Design review of the part built by this model. Coordinates are the model's own, in mm. A direction names the side the tool comes from. Give positions to 0.01 mm unless a question says otherwise; leave off trailing zeros. Order: outer loops, then holes, each group sorted by start corner. A loop starts at its lowest first (then second) coordinate and runs counter-clockwise, first axis right, second up. Notation, with made-up numbers: (45.5, -26) -> (93.5, -26) arc R32 cw to (93.5, 8) -> close; hole circle Ø4 at (-3, 78). An arc over 180 degrees is marked (long way). One line per item, written item: value. Start each with the question number.
1) Consider section A-A (x = 29). State the section outline as (y, z) points.
2) Tool access review of faces 1 (the face through (-40, 4, 0)), 2 (the face through (-37, 7, -26)), 3 (the face through (-1, 4, -27.5)), 4 (the face through (-1, 4, 27.5)), 5 (the face through (35, 3, 0)): name each direction out of +Z, -Z, +X, -X, +Y, -Y from which nothing blocks a thin tool from reaching the whole face with its end or side.
3) For pin 1 (2.5 mm diameter, centred on y = 3, z = 4.5, fed in from +X); pin 2 (1 mm diameter, centred on y = 3.5, z = -16, fed in from +X); pin 3 (3 mm diameter, centred on x = -2, y = 6, fed in from -Z); pin 4 (1 mm diameter, centred on y = 6.5, z = 26.5, fed in from -X), all flat-tipped, find the tip position at first contact; note any pin that passes through.
4) Consider section C-C (x = -55.5). State the section outline as (y, z) points.
5) The part is to be moulded in two halves that separate along X. For faces 6 (the face through (0, 3, 22.5)), 7 (the face through (37, 7, 26)), 8 (the face through (40, 4, 0)), say which applies: released by +X, released by -X, zero draft, split by the parting line, or undercut.
6) Wall thickness on line 1 along X through (y, z) = (1.75, -20); line 2 along X through (y, z) = (5.25, -26); line 3 along Z through (x, y) = (-31.5, 2.25): over which ranges is each line inside the solid? List them lowest first. Write a range as from..to.
7) Consider section B-B (z = 5). State the section outline as (x, y) points, plus the area to 3 significant figures.
from build123d import *

# Parameters (mm, degrees)
SKETCH1_W           = 132
SKETCH1_H           = 87
BOSS_EXTRUDE1_DEPTH = 2
SKETCH2_W           = 80
SKETCH2_H           = 55
BOSS_EXTRUDE2_DEPTH = 5
SKETCH3_W           = 76
SKETCH3_H           = 51
CUT_EXTRUDE1_DEPTH  = 2
CUT_EXTRUDE2_REACH  = 7
SKETCH4_W           = 70
SKETCH4_H           = 45
SKETCH5_W           = 2
SKETCH5_H           = 41
SKETCH5_W_2         = 66
SKETCH5_H_2         = 2
CUT_EXTRUDE3_DEPTH  = 2
CUT_EXTRUDE4_DEPTH  = 2


with BuildPart() as part:
    # Sketch1 → Boss-Extrude1 (new body)
    with BuildSketch(Plane(origin=(0, 0, 0), x_dir=(1, 0, 0), z_dir=(0, 1, 0))):
        Rectangle(SKETCH1_W, SKETCH1_H)
    extrude(amount=BOSS_EXTRUDE1_DEPTH)

    # Sketch2 → Boss-Extrude2 (add)
    with BuildSketch(Plane(origin=(0, 2, 0), x_dir=(1, 0, 0), z_dir=(0, 1, 0))):
        Rectangle(SKETCH2_W, SKETCH2_H)
    extrude(amount=BOSS_EXTRUDE2_DEPTH)

    # Sketch3 → Cut-Extrude1 (cut)
    with BuildSketch(Plane(origin=(0, 7, 0), x_dir=(1, 0, 0), z_dir=(0, 1, 0))):
        Rectangle(SKETCH3_W, SKETCH3_H)
    extrude(amount=-CUT_EXTRUDE1_DEPTH, mode=Mode.SUBTRACT)

    # Sketch4 → Cut-Extrude2 (cut, up to next)
    with BuildSketch(Plane(origin=(0, 5, 0), x_dir=(1, 0, 0), z_dir=(0, 1, 0)), mode=Mode.PRIVATE) as cut_extrude2_sk1:
        Rectangle(SKETCH4_W, SKETCH4_H)
    cut_extrude2_tool1 = extrude(cut_extrude2_sk1.sketch, amount=-CUT_EXTRUDE2_REACH, mode=Mode.PRIVATE) & part.part
    add(cut_extrude2_tool1.solids().sort_by_distance((0, 5, 0))[0], mode=Mode.SUBTRACT)

    # Sketch5 → Cut-Extrude3 (cut)
    with BuildSketch(Plane(origin=(0, 7, 0), x_dir=(1, 0, 0), z_dir=(0, 1, 0))):
        with Locations((-39, 0)):
            Rectangle(SKETCH5_W, SKETCH5_H)
        with Locations((39, 0)):
            Rectangle(SKETCH5_W, SKETCH5_H)
        with Locations((0, 26.5)):
            Rectangle(SKETCH5_W_2, SKETCH5_H_2)
        with Locations((0, -26.5)):
            Rectangle(SKETCH5_W_2, SKETCH5_H_2)
    extrude(amount=-CUT_EXTRUDE3_DEPTH, mode=Mode.SUBTRACT)

    # Sketch6 → Cut-Extrude4 (cut)
    with BuildSketch(Plane(origin=(0, 2, 0), x_dir=(1, 0, 0), z_dir=(0, 1, 0))):
        with BuildLine():
            Line((-12.085608445, 43.5), (12.085608445, 43.5))
            ThreePointArc((12.085608445, 43.5), (0, 31.414391555), (-12.085608445, 43.5))
        make_face()
    extrude(amount=-CUT_EXTRUDE4_DEPTH, mode=Mode.SUBTRACT)


solid = part.part
Checked values:
1. outline: (0, -43.5) -> (2, -43.5) -> (2, -27.5) -> (5, -27.5) -> (5, -22.5) -> (0, -22.5) -> close; (0, 22.5) -> (5, 22.5) -> (5, 27.5) -> (2, 27.5) -> (2, 43.5) -> (0, 43.5) -> close
2. face 1: +Z, -Z, -X, +Y
2. face 2: +Z, -Z, +X, -X, +Y
2. face 3: -Z, +X, -X, +Y
2. face 4: +Z, +X, -X, +Y
2. face 5: +Y, -Y
3. pin 1: stops at x = 66
3. pin 2: stops at x = 40
3. pin 3: stops at z = -27.5
3. pin 4: stops at x = -40
4. outline: (0, -43.5) -> (2, -43.5) -> (2, 43.5) -> (0, 43.5) -> close
5. face 6: undercut
5. face 7: zero draft
5. face 8: released by +X
6. line 1: x = -66..-35, 35..66
6. line 2: x = -40..-33, 33..40
6. line 3: z = -27.5..-22.5, 22.5..27.5
7. outline: (-66, 0) -> (-35, 0) -> (-35, 5) -> (-40, 5) -> (-40, 2) -> (-66, 2) -> close; (35, 0) -> (66, 0) -> (66, 2) -> (40, 2) -> (40, 5) -> (35, 5) -> close
7. area: 154 mm^2
